```python
from build123d import *

# Parameters (mm, degrees)
BOSS_EXTRUDE1_DEPTH                           = 10.668
CSK_FOR_2_FLAT_HEAD_MACHINE_SCREW1_AT_2_COUNT = 2
CSK_FOR_2_FLAT_HEAD_MACHINE_SCREW1_AT_2_PITCH = 28.241625
CSK_FOR_2_FLAT_HEAD_MACHINE_SCREW1_AT_3_COUNT = 2
CSK_FOR_2_FLAT_HEAD_MACHINE_SCREW1_AT_3_PITCH = 24.18748446
SKETCH4_R                                     = 6.477
CUT_EXTRUDE1_DEPTH                            = 1.5748
SKETCH5_R                                     = 4.7879
CUT_EXTRUDE2_DEPTH                            = 11.668
SKETCH6_W                                     = 8.0264
SKETCH6_H                                     = 10.033
CUT_EXTRUDE3_DEPTH                            = 5.08
DRAFT2_ANGLE                                  = 45
CHAMFER1_SIZE                                 = 3.175
CHAMFER2_SIZE                                 = 6.35
CUT_EXTRUDE4_DEPTH                            = 2.7432


with BuildPart() as part:
    # Sketch1 → Boss-Extrude1 (new body)
    with BuildSketch(Plane.XY):
        Polygon((21.463, 6.6802), (-18.288, 6.6802), (-18.288, -6.6802), (-6.6802, -6.6802), (-6.6802, -23.495), (6.6802, -23.495), (6.6802, -6.6802), (21.463, -6.6802), align=None)
    extrude(amount=BOSS_EXTRUDE1_DEPTH)

    # Sketch3 → CSK for #2 Flat Head Machine Screw1 (revolve, cut)
    with BuildSketch(Plane(origin=(15.859125, 0, 10.668), x_dir=(0, -1, 0), z_dir=(1, 0, 0))):
        Polygon((0, 0), (0, 10.668), (1.2192, 10.668), (1.2192, 3.853535587), (2.1844, 2.7432), (2.1844, 0), align=None)
    csk_for_2_flat_head_machine_screw1 = revolve(axis=Axis((15.859125, 0, 17.018), (0, 0, -1)), mode=Mode.SUBTRACT)

    # CSK for #2 Flat Head Machine Screw1 at 2: CSK for #2 Flat Head Machine Screw1 ×2
    with Locations(*[(-i * CSK_FOR_2_FLAT_HEAD_MACHINE_SCREW1_AT_2_PITCH, 0, 0) for i in range(1, CSK_FOR_2_FLAT_HEAD_MACHINE_SCREW1_AT_2_COUNT)]):
        add(csk_for_2_flat_head_machine_screw1, mode=Mode.SUBTRACT)

    # CSK for #2 Flat Head Machine Screw1 at 3: CSK for #2 Flat Head Machine Screw1 ×2
    with Locations(*[Vector(-0.65567484, -0.755043379, 0) * (i * CSK_FOR_2_FLAT_HEAD_MACHINE_SCREW1_AT_3_PITCH) for i in range(1, CSK_FOR_2_FLAT_HEAD_MACHINE_SCREW1_AT_3_COUNT)]):
        add(csk_for_2_flat_head_machine_screw1, mode=Mode.SUBTRACT)

    # Sketch4 → Cut-Extrude1 (cut)
    with BuildSketch(Plane.XY.offset(10.668)):
        Circle(SKETCH4_R)
    extrude(amount=-CUT_EXTRUDE1_DEPTH, mode=Mode.SUBTRACT)

    # Sketch5 → Cut-Extrude2 (cut, through all)
    with BuildSketch(Plane.XY.offset(10.668)):
        Circle(SKETCH5_R)
    extrude(amount=-CUT_EXTRUDE2_DEPTH, mode=Mode.SUBTRACT)

    # Sketch6 → Cut-Extrude3 (cut)
    with BuildSketch(Plane(origin=(0, 0, 0), x_dir=(-1, 0, 0), z_dir=(0, 0, -1))):
        with Locations((-6.24205, 10.483214746)):
            Rectangle(SKETCH6_W, SKETCH6_H)
    extrude(amount=-CUT_EXTRUDE3_DEPTH, mode=Mode.SUBTRACT)

    # Draft2
    draft2_faces = [part.faces().sort_by_distance(p)[0] for p in [
        (6.24205, 6.073457373, 5.08),
    ]]
    draft(draft2_faces, Plane(origin=(10.25525, 5.466714746, 5.08), x_dir=(1, 0, 0), z_dir=(0, 1, 0)), DRAFT2_ANGLE)

    # Chamfer1
    chamfer1_edges = [part.edges().sort_by_distance(p)[0] for p in [
        (21.463, -6.6802, 5.334),
        (6.6802, -23.495, 5.334),
        (-6.6802, -23.495, 5.334),
        (-18.288, -6.6802, 5.334),
        (-18.288, 6.6802, 5.334),
        (21.463, 6.6802, 5.334),
    ]]
    chamfer(chamfer1_edges, length=CHAMFER1_SIZE)

    # Chamfer2
    chamfer2_edges = [part.edges().sort_by_distance(p)[0] for p in [
        (6.6802, -6.6802, 5.334),
        (-6.6802, -6.6802, 5.334),
    ]]
    chamfer(chamfer2_edges, length=CHAMFER2_SIZE)

    # Sketch7 → Cut-Extrude4 (cut)
    with BuildSketch(Plane.XY.offset(10.668)):
        with BuildLine():
            Line((3.7719, -13.69343597), (6.675135951, -10.790200019))
            Line((6.675135951, -10.790200019), (3.260798724, -7.375862792))
            ThreePointArc((3.260798724, -7.375862792), (0, -8.0645), (-3.260798724, -7.375862792))
            Line((-3.260798724, -7.375862792), (-6.675135951, -10.790200019))
            Line((-6.675135951, -10.790200019), (-3.7719, -13.69343597))
            Line((-3.7719, -13.69343597), (-3.7719, -18.2626))
            ThreePointArc((-3.7719, -18.2626), (0, -22.0345), (3.7719, -18.2626))
            Line((3.7719, -18.2626), (3.7719, -13.69343597))
        make_face()
        with BuildLine():
            Line((12.37263597, -5.0927), (17.63043597, -5.0927))
            Line((17.63043597, -5.0927), (19.8755, -2.84763597))
            Line((19.8755, -2.84763597), (19.8755, 2.84763597))
            Line((19.8755, 2.84763597), (17.63043597, 5.0927))
            Line((17.63043597, 5.0927), (8.0645, 5.0927))
            Line((8.0645, 5.0927), (8.0645, 0))
            ThreePointArc((8.0645, 0), (7.500371575, -2.963205441), (5.886910197, -5.511846205))
            Line((5.886910197, -5.511846205), (8.920199981, -8.545135989))
            Line((8.920199981, -8.545135989), (12.37263597, -5.0927))
        make_face()
        with BuildLine():
            Line((-14.45543597, 5.0927), (-16.7005, 2.84763597))
            Line((-16.7005, 2.84763597), (-16.7005, -2.84763597))
            Line((-16.7005, -2.84763597), (-14.45543597, -5.0927))
            Line((-14.45543597, -5.0927), (-12.37263597, -5.0927))
            Line((-12.37263597, -5.0927), (-8.920199981, -8.545135989))
            Line((-8.920199981, -8.545135989), (-5.886910197, -5.511846205))
            ThreePointArc((-5.886910197, -5.511846205), (-7.500371575, -2.963205441), (-8.0645, 0))
            Line((-8.0645, 0), (-8.0645, 5.0927))
            Line((-8.0645, 5.0927), (-14.45543597, 5.0927))
        make_face()
    extrude(amount=-CUT_EXTRUDE4_DEPTH, mode=Mode.SUBTRACT)


solid = part.part
```
Could you check a few things on this model? Use its own coordinates, in mm. A direction names the side the tool comes from. Coordinates: 2 decimals unless noted, no trailing zeros. Loops run counter-clockwise (first coordinate to the right, second up) from the corner with the lowest first, then second, coordinate; pieces in that order, holes last.
1) Imagine slicing it at A-A (x = 0). State how many separate pieces and enclosed holes the cut face has, and give its area (3 significant figures).
Reported:
separate pieces: 3
enclosed holes: 0
area: 156 mm2
2) Imagine slicing it at D-D (y = -9.5). List the corners of the cut face in (x, z) for me.
Reported:
outline: (-10.21, 0) - (10.21, 0) - (10.21, 10.67) - (5.38, 10.67) - (5.38, 7.92) - (-5.38, 7.92) - (-5.38, 10.67) - (-10.21, 10.67) - close
3) Imagine slicing it at B-B (y = -15). List the corners of the cut face in (x, z) for me.
Reported:
outline: (-6.68, 0) - (6.68, 0) - (6.68, 10.67) - (3.77, 10.67) - (3.77, 7.92) - (-3.77, 7.92) - (-3.77, 10.67) - (-6.68, 10.67) - close
4) Imagine slicing it at C-C (x = 9.5). List the corners of the cut face in (y, z) for me, and give its area (3 significant figures).
Reported:
outline: (-10.21, 0) - (5.47, 0) - (5.47, 5.08) - (6.68, 6.29) - (6.68, 10.67) - (5.09, 10.67) - (5.09, 7.92) - (-7.97, 7.92) - (-7.97, 10.67) - (-10.21, 10.67) - close
area: 137 mm2
5) Please list where these lines run through material, in increasing order: line 1 along Y through (x, z) = (0, 6.75) (3 decimals); line 2 along X through (y, z) = (-16, 9.75); line 3 along Y through (x, z) = (2, 10.25) (3 decimals).
Reported:
line 1: y = -23.495 to -19.482, -17.043 to -4.788, 4.788 to 6.68
line 2: x = -6.68 to -3.77, 3.77 to 6.68
line 3: y = -23.495 to -21.461, -7.813 to -6.16, 6.16 to 6.68
6) Thinking about a two-plate mould opening in Y: for faces 1 (the face through (9.81, -9.9, 5.26)), 2 (the face through (-16.7, 0, 9)), 3 (the face through (10.255, 6, 3)), 4 (the face through (-15.594, -3.954, 9.316)), which applies, released by +Y, released by -Y, zero draft, split by the parting line, or undercut?
Reported:
face 1: released by -Y
face 2: undercut
face 3: zero draft
face 4: undercut
7) Which directions (+Z, -Z, +X, -X, +Y, -Y) give clear straight access to the entire face, cutting with the end or side of a thin tool? Please do faces 5 (the face through (-6.68, -17, 5)), 6 (the face through (1, -5, 0)), 7 (the face through (-7.425, -7.05, 9.316)).
Reported:
face 5: +Z, -Z, -X, -Y
face 6: -Z, +X, -X, +Y, -Y
face 7: +Z
8) Will these pins go through, and if not, where does the flat tip stop? pin 1 Ø1 at (x, z) = (9.5, 4.5) entering from +Y; pin 2 Ø2 at (y, z) = (-11.5, 4) entering from -X; pin 3 Ø5 at (y, z) = (-10.5, 4) entering from -X; pin 4 Ø1.5 at (x, y) = (0, -18.26) entering from +Z.
Reported:
pin 1: stops at y = 5.47
pin 2: stops at x = -9.21
pin 3: stops at x = -11.71
pin 4: passes through
